Autodesk Inventor part; units mm, degrees
ref_plane "YZ Plane" through (0, 0, 0) normal (1, 0, 0) x (0, 1, 0)
ref_plane "XZ Plane" through (0, 0, 0) normal (0, 1, 0) x (-1, 0, 0)
ref_plane "XY Plane" through (0, 0, 0) normal (0, 0, 1) x (1, 0, 0)
sketch "Sketch1" plane through (0, 0, 0) normal (1, 0, 0) x (0, 1, 0)
  circle A0 centre (0, 0) radius 20
  line L0 (8.5, 8.5) -> (-16.9, 8.5)
  line L1 (8.5, 8.5) -> (8.5, -16.9)
  line L2 (0, 0) -> (0, 20)
  line L3 (0, 20) -> (-60.9241, 20)
  line L4 (-60.9241, 20) -> (-60.9241, 18.5)
  line L5 (-60.9241, 18.5) -> (0, 18.5)
  line L6 (0, 18.5) -> (0, 20)
  line L7 (0, 0) -> (14.1421, 14.1421)
  line L8 (0, 0) -> (20, 0)
  line L9 (-16.9, 8.5) -> (-16.9, 18.5)
  line L10 (-16.9, 8.5) -> (-22.9, 14.5)
  line L11 (-22.9, 14.5) -> (-22.9, 18.5)
  line L12 (12.3744, 12.3744) -> (12.1502, 13.2109)
  line L13 (11.3137, 13.435) -> (9.2071, 11.3284)
  line L14 (9.4313, 10.4919) -> (10.2678, 10.2678)
  line L15 (8.5, 8.5) -> (8.5, -16.9)
  line L16 (20, 0) -> (20, -60.9241)
  line L17 (20, -60.9241) -> (18.5, -60.9241)
  line L18 (18.5, -60.9241) -> (18.5, 0)
  line L19 (8.5, -16.9) -> (18.5, -16.9)
  line L20 (8.5, -16.9) -> (14.5, -22.9)
  line L21 (14.5, -22.9) -> (18.5, -22.9)
  arc A1 (9.2071, 11.3284) -> (9.4313, 10.4919) centre (9.5607, 10.9749) ccw
  arc A2 (12.1502, 13.2109) -> (11.3137, 13.435) centre (11.6673, 13.0815) ccw
  line L22 (10.4311, 10.4311) -> (9.483, 10.6851)
  arc A3 (9.3485, 11.187) -> (9.483, 10.6851) centre (9.5607, 10.9749) ccw
  line L23 (9.3485, 11.187) -> (11.4551, 13.2936)
  arc A4 (11.957, 13.1591) -> (11.4551, 13.2936) centre (11.6673, 13.0815) ccw
  line L24 (11.957, 13.1591) -> (12.2111, 12.2111)
  point P0 (0, 8.5)
  point P1 (-17.7041, 9.3041)
  point P2 (-16.9, 10.6953)
  dimension "d0" = 40
  dimension "d1" = 25.4
  dimension "d2" = 1.5
  dimension "d4" = 45
  dimension "d6" = 45
  dimension "d7" = 4
  dimension "d8" = 10
  dimension "d10" = 2.5
  dimension "d11" = 2.5
  dimension "d12" = 60
  dimension "d13" = 1.5
  dimension "d15" = 0.5
  dimension "d16" = 0.2
extrude "Extrusion1" add sketch "Sketch1" along normal blind 238.3 contours L7 L12 A2 L13 A1 L14 L0 L2 A0 | L7 L24 A4 L23 A3 L22 L14 A1 L13 A2 L12 | L5 L2 L0 L9 A0 | A0 L9 L5 | L7 L22 A3 L23 A4 L24 | L9 L10 A0 | A0 L10 L11 L5 L9
sketch "Sketch2" plane through (0, -22.9, 18.5) normal (0, 0, 1) x (1, 0, 0)
  line L0 (0, 22.9) -> (0, 0)
  line L1 (0, 0) -> (238.3, 0)
  line L2 (238.3, 22.9) -> (238.3, 0)
  line L3 (0, 22.9) -> (238.3, 22.9)
  line L4 (38.3257, 13.1) -> (36.6514, 16)
  line L5 (36.6514, 16) -> (38.3257, 18.9)
  line L6 (38.3257, 18.9) -> (41.6743, 18.9)
  line L7 (41.6743, 18.9) -> (43.3486, 16)
  line L8 (43.3486, 16) -> (41.6743, 13.1)
  line L9 (41.6743, 13.1) -> (38.3257, 13.1)
  line L10 (0, 6) -> (238.3, 6)
  circle A0 centre (40, 16) radius 1.65
  dimension "d20" = 10
  dimension "d21" = 5.8
  dimension "d22" = 40
  dimension "d25" = 3.3
extrude "Extrusion2" cut sketch "Sketch2" against normal blind 6 contours L4 L5 L6 L7 L8 L9 | A0
extrude "Extrusion3" cut sketch "Sketch2" against normal through all contours A0
sketch "Sketch3" plane through (0, -22.9, 18.5) normal (0, 0, 1) x (1, 0, 0)
  line L0 (0, 37.0421) -> (238.3, 37.0421)
  line L1 (0, 0) -> (238.3, 0)
  line L2 (0, 22.9) -> (0, 0)
  line L3 (0, 22.9) -> (0, 37.0421)
  line L4 (2.4384, 37.0421) -> (17.8575, 0)
  line L5 (0, 0) -> (238.3, 0)
  line L6 (2.4384, 37.0421) -> (0, 42.9)
  point P0 (0, 26.9698)
  dimension "d28" = 112.6
sketch "Sketch4" plane through (238.3, 14.1421, 14.1421) normal (0, 0.7071, -0.7071) x (-1, 0, 0)
  line L0 (238.3, 0) -> (0, 0)
  line L1 (0, -7.9792) -> (0, 0)
  line L2 (238.3, -7.9792) -> (0, -7.9792)
  circle A0 centre (208.3, -4) radius 1.5
  line L3 (238.3, -7.9792) -> (238.3, 0)
  line L4 (119.15, -7.9792) -> (119.15, 0)
  ellipse E0 centre (198.3, -18.8686) end of major axis (196.65, -18.8686) minor radius 1.1667
  point P0 (238.3, -20)
  dimension "d34" = 3
  dimension "d35" = 4
  dimension "d46" = 30
extrude "Extrusion5" cut sketch "Sketch4" against normal blind 3 contours A0
ref_plane "Work Plane1" through (119.15, 0, 0) normal (-1, 0, 0) x (0, 0, 1)
mirror "Mirror1" about plane through (119.15, 0, 0) normal (-1, 0, 0) of "Extrusion5", "Extrusion2", "Extrusion3"
sketch "Sketch6" plane through (238.3, 0, 0) normal (1, 0, 0) x (0, 0, -1)
  line L0 (-14.5, -22.9) -> (-8.5, -16.9)
  line L1 (-8.5, -16.9) -> (-8.5, 8.5)
  line L2 (-8.5, 8.5) -> (-14.1421, 14.1421)
  arc A0 (-14.1421, 14.1421) -> (-20, 0) centre (0, 0) ccw
  line L3 (-20, 0) -> (-18.5, 0)
  line L4 (-18.5, 0) -> (-18.5, -22.9)
  line L5 (-18.5, -22.9) -> (-14.5, -22.9)
  line L6 (-18.5, -22.9) -> (-18.4, -22.9)
  line L7 (-18.4, -22.9) -> (-18.4, 0)
  line L8 (-18.4, 0) -> (-18.5, 0)
  line L9 (-18.5, 0) -> (-18.5, -22.9)
  dimension "d50" = 0.1
extrude "Extrusion7" cut sketch "Sketch6" against normal through all contours L5 L4 L8 L7
properties part number "ESQUINA_REDONDEADA_R20" material "Steel, Mild, Welded"
CAD build for the part. Positions are in the model's coordinates, mm. A direction names the side the tool comes from. Give positions to 0.01 mm unless a question says otherwise; leave off trailing zeros. Order: outer loops, then holes, each group sorted by start corner. A loop starts at its lowest first (then second) coordinate and runs counter-clockwise, first axis right, second up.
(1) Mould opens along X. For faces 1 (the cylindrical face through (209.73, 9.95, 12.04)), 2 (the cylindrical face through (117.5, 7.6, 18.5)) say: released by +X, released by -X, zero draft, split by the parting line, or undercut.
(2) Saw through at C-C, the plane y = -20. Give the cut face in (x, z), then the cut area to 3 significant figures.
(3) Tool access for faces 3 (the flat face through (200, -6, 12.5)), 4 (the cylindrical face through (28.57, 10.59, 12.68)), 5 (the flat face through (121, -12, 18.4)): list every direction of +Z, -Z, +X, -X, +Y, -Y with a clear straight run to the whole face (end or side of a thin tool).
(4) Flat gauge pins, fed straight in: pin 1 (1 mm diameter, centred on x = 73.5, z = 12, fed in from +Y); pin 2 (1.5 mm diameter, centred on x = 102, z = 11, fed in from +Y); pin 3 (2.5 mm diameter, centred on x = 40.5, z = 16.5, fed in from +Y). Where does each tip first touch, or does it go through?
(5) Saw through at B-B, the plane z = 16.25. Give the cut face in (x, y), then the cut area to 3 significant figures.
(6) Drill centre lines: L1, parallel to Z at x = 166.5, y = -6; L2, parallel to Y at x = 40, z = 11.25; L3, parallel to Y at x = 40, z = 11.4. Where is each one in solid material? Low to high.
(7) Saw through at A-A, the plane x = 96. Give the cut face in (y, z), then the cut area to 3 significant figures.
Results found:
1. face 1: undercut
1. face 2: zero draft
2. outline: (0, 11.6) - (238.3, 11.6) - (238.3, 18.4) - (0, 18.4) - close
2. area: 1,620 mm2
3. face 3: +Z
3. face 4: none
3. face 5: +Z, +X, -X, -Y
4. pin 1: stops at y = 12.5
4. pin 2: stops at y = 11.75
4. pin 3: stops at y = 12.94
5. outline: (0, -22.9) - (238.3, -22.9) - (238.3, 11.66) - (0, 11.66) - close; hole (36.65, -6.9) - (38.33, -9.8) - (41.67, -9.8) - (43.35, -6.9) - (41.67, -4) - (38.33, -4) - close; hole (194.95, -6.9) - (196.63, -9.8) - (199.97, -9.8) - (201.65, -6.9) - (199.97, -4) - (196.63, -4) - close
5. area: 8,180 mm2
6. L1: z = 8.5 to 18.4
6. L2: y = -19.65 to -8.55, -5.25 to 11.25
6. L3: y = -19.8 to -8.55, -5.25 to 11.4
7. outline: (-22.9, 14.5) - (-16.9, 8.5) - (8.5, 8.5) - (14.14, 14.14) arc R20 ccw to (0, 20) - (0, 18.4) - (-22.9, 18.4) - close
7. area: 330 mm2
